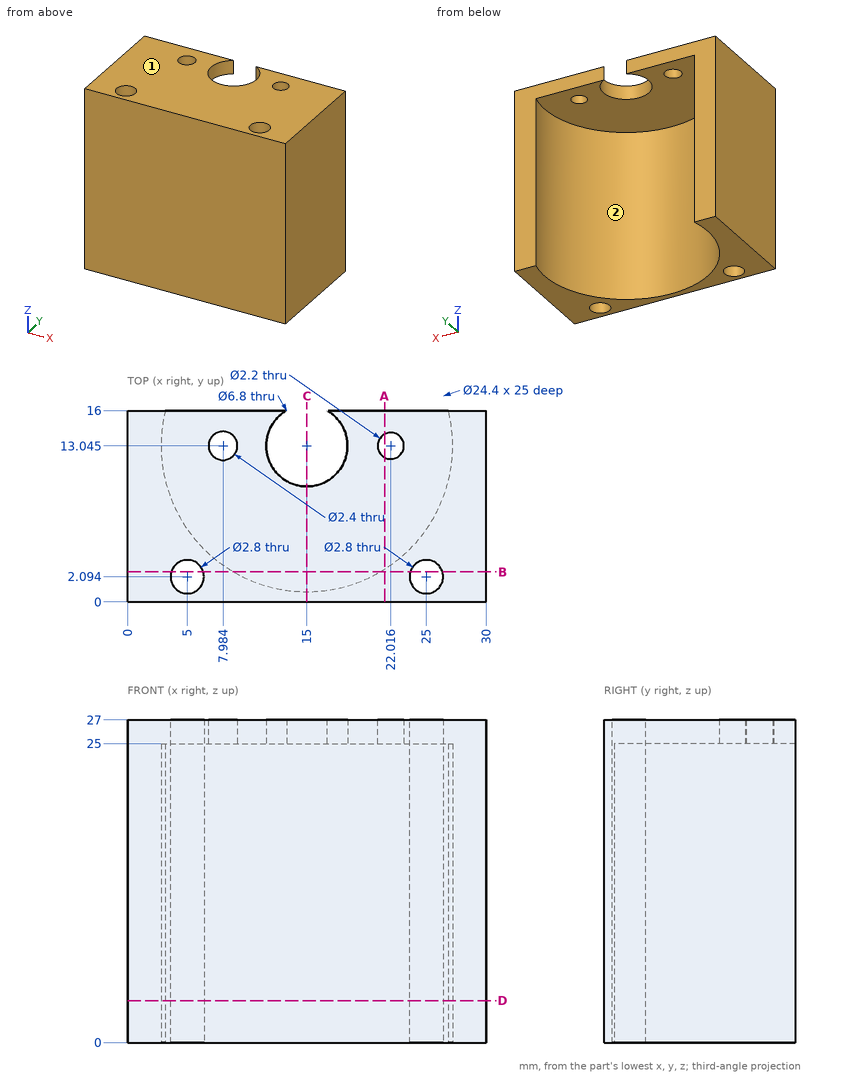
Part print with two shaded views. Sizes in mm from the minimum x, y, z corner. A direction names the side the tool comes from. Round coordinates to 2 decimals unless told otherwise and drop trailing zeros. Write each loop counter-clockwise with the first axis right and the second up, starting at its lowest first coordinate (ties: lowest second). Pieces come first, ordered by that corner, then holes. Notation, with made-up numbers: (29, 86) -> (55, 86) arc R22 cw to (55, 112) -> close; hole circle Ø6 at (53.5, 10.25). An arc over 180 degrees is marked (long way). Put each result on its own line as item: value.
Item 1: Wall check: probe 1 along X at (y, z) = (13, 17.25); probe 2 along Z at (x, y) = (14.5, 6.5); probe 3 along X at (y, z) = (11.5, 17). Give the ranges that are in metal, low to high. Write a range as from..to.
Here are the results:
probe 1: x = 0..2.8, 27.2..30
probe 2: z = 25..27
probe 3: x = 0..2.9, 27.1..30
Item 2: Slice it at A-A, the plane x = 21.5. Give the cut face in (y, z).
Here are the results:
outline: (0, 0) -> (2.72, 0) -> (2.72, 25) -> (12.07, 25) -> (12.07, 27) -> (0, 27) -> close; (14.02, 25) -> (16, 25) -> (16, 27) -> (14.02, 27) -> close
Item 3: Slice it at C-C, the plane x = 15. Give the cut face in (y, z) (1 decimal).
Here are the results:
outline: (0, 0) -> (0.8, 0) -> (0.8, 25) -> (9.6, 25) -> (9.6, 27) -> (0, 27) -> close
Item 4: Slice it at D-D, the plane z = 3.5. Give the cut face in (x, y) (1 decimal).
Here are the results:
outline: (0, 0) -> (30, 0) -> (30, 16) -> (26.8, 16) arc R12.2 cw (long way) to (3.2, 16) -> (0, 16) -> close; hole circle Ø2.8 at (5, 2.1); hole circle Ø2.8 at (25, 2.1)
Item 5: Slice it at B-B, the plane y = 2.5. Give the cut face in (x, z) (1 decimal).
Here are the results:
outline: (0, 0) -> (3.7, 0) -> (3.7, 27) -> (0, 27) -> close; (6.3, 0) -> (8.9, 0) -> (8.9, 25) -> (21.1, 25) -> (21.1, 0) -> (23.7, 0) -> (23.7, 27) -> (6.3, 27) -> close; (26.3, 0) -> (30, 0) -> (30, 27) -> (26.3, 27) -> close
Item 6: Flat gauge pins, fed straight in: P1, Ø4.5, axis at x = 16.5, y = 6.5, coming from the -Z side; P2, Ø6, axis at x = 12.5, z = 12.5, coming from the +Y side (1 decimal); P3, Ø3, axis at x = 20.5, z = 18, coming from the +Y side. Where does each tip first touch, or does it go through?
Here are the results:
P1: stops at z = 25
P2: stops at y = 2.2
P3: stops at y = 3.05
Item 7: Tool access for the marked faces 1 and 2: list every direction of +Z, -Z, +X, -X, +Y, -Y with a clear straight run to the whole face (end or side of a thin tool).
Here are the results:
face 1: +Z, +X, -X, +Y, -Y
face 2: -Z
